from build123d import *

# Parameters (mm, degrees)
F0_R     = 53.975
F0_R_2   = 19.05
F0_R_3   = 12.7
F1_DEPTH = 12.7
F2_DEPTH = 50.8
F3_R     = 5.08
F4_SIZE  = 1.016


with BuildPart() as f1:
    # F0 (on Front) → F1 (new body)
    with BuildSketch(Plane.XZ):
        Circle(F0_R)
        with BuildLine():
            ThreePointArc((7.835162, 38.906399), (28.0633, 28.0633), (38.906399, 7.835162))
            ThreePointArc((38.906399, 7.835162), (44.971887, 5.837391), (47.5615, 0))
            ThreePointArc((47.5615, 0), (44.971887, -5.837391), (38.906399, -7.835162))
            ThreePointArc((38.906399, -7.835162), (28.0633, -28.0633), (7.835162, -38.906399))
            ThreePointArc((7.835162, -38.906399), (7.864284, -39.296467), (7.874, -39.6875))
            ThreePointArc((7.874, -39.6875), (-0.391033, -47.551784), (-7.835162, -38.906399))
            ThreePointArc((-7.835162, -38.906399), (-28.0633, -28.0633), (-38.906399, -7.835162))
            ThreePointArc((-38.906399, -7.835162), (-47.5615, 0), (-38.906399, 7.835162))
            ThreePointArc((-38.906399, 7.835162), (-28.0633, 28.0633), (-7.835162, 38.906399))
            ThreePointArc((-7.835162, 38.906399), (-0.391033, 47.551784), (7.874, 39.6875))
            ThreePointArc((7.874, 39.6875), (7.864284, 39.296467), (7.835162, 38.906399))
        make_face(mode=Mode.SUBTRACT)
        with BuildLine():
            ThreePointArc((38.906399, -7.835162), (31.8135, 0), (38.906399, 7.835162))
            ThreePointArc((38.906399, 7.835162), (28.0633, 28.0633), (7.835162, 38.906399))
            ThreePointArc((7.835162, 38.906399), (0, 31.8135), (-7.835162, 38.906399))
            ThreePointArc((-7.835162, 38.906399), (-28.0633, 28.0633), (-38.906399, 7.835162))
            ThreePointArc((-38.906399, 7.835162), (-33.850109, 5.284387), (-31.8135, 0))
            ThreePointArc((-31.8135, 0), (-33.850109, -5.284387), (-38.906399, -7.835162))
            ThreePointArc((-38.906399, -7.835162), (-28.0633, -28.0633), (-7.835162, -38.906399))
            ThreePointArc((-7.835162, -38.906399), (0, -31.8135), (7.835162, -38.906399))
            ThreePointArc((7.835162, -38.906399), (28.0633, -28.0633), (38.906399, -7.835162))
        make_face()
        Circle(F0_R_2, mode=Mode.SUBTRACT)
        Circle(F0_R_2)
        Circle(F0_R_3, mode=Mode.SUBTRACT)
    extrude(amount=F1_DEPTH)

    # F0 (on Front) → F2 (join)
    with BuildSketch(Plane.XZ):
        Circle(F0_R_2)
        Circle(F0_R_3, mode=Mode.SUBTRACT)
    extrude(amount=F2_DEPTH)

    # F3
    f3_edges = [f1.edges().sort_by_distance(p)[0] for p in [
        (-19.05, -12.7, 0),
    ]]
    fillet(f3_edges, radius=F3_R)

    # F4
    f4_edges = [f1.edges().sort_by_distance(p)[0] for p in [
        (53.975, -6.35, 0),
        (-53.975, 0, 0),
        (-53.975, -12.7, 0),
        (-40.468601, 0, -7.835162),
        (-38.906399, -6.35, 7.835162),
        (-40.468601, -12.7, -7.835162),
        (-7.835162, -6.35, -38.906399),
        (7.835162, 0, -40.468601),
        (7.835162, -12.7, -40.468601),
        (38.906399, -6.35, -7.835162),
        (40.468601, 0, 7.835162),
        (40.468601, -12.7, 7.835162),
        (7.874, -6.35, 39.6875),
        (-7.874, 0, 39.6875),
        (-7.874, -12.7, 39.6875),
        (-19.05, -50.8, 0),
        (-12.7, 0, 0),
        (12.7, -25.4, 0),
        (-12.7, -50.8, 0),
    ]]
    chamfer(f4_edges, length=F4_SIZE)


solid = f1.part
Input: part model. Units: mm. Frame: model coordinates. A direction names the side the tool comes from. Give positions to 0.01 mm unless a question says otherwise; leave off trailing zeros. Loops run counter-clockwise (first coordinate to the right, second up) from the corner with the lowest first, then second, coordinate; pieces in that order, holes last. Notation, with made-up numbers: (56, -29.5) -> (93, -29.5) arc R27 ccw to (93, -8.5) -> close; hole circle Ø3 at (45.5, 46). An arc over 180 degrees is marked (long way). Answer as a JSON object with one key per item and string values. Group by question number.
Item 1: Reachability of faces 1 (the cylindrical face through (-15.12, -33.56, -11.59)), 2 (the flat face through (12, -50.8, 7)) from +Z, -Z, +X, -X, +Y, -Y: full face, straight path, thin tool, end or side. Return the list, or none.
Item 2: Cut plane B-B, the plane z = 4. State how many separate pieces and enclosed holes the cut face has, and give its area (3 significant figures).
Item 3: Cut plane A-A, the plane y = -36.5. Return the cut outline in (x, z), and give its area (3 significant figures).
Item 4: Line query: probe 1 along Z at (x, y) = (0, -10.5) (1 decimal); probe 2 along Z at (x, y) = (-2, -10); probe 3 along Y at (x, z) = (-34.5, -31.5). Output: solid intervals per line, ascending.
Item 5: Pull-direction query (X, two-part tool) for faces 3 (the cylindrical face through (-39.78, -6.28, 36.48)), 4 (the cylindrical face through (-2.75, -25.06, -12.4)), 5 (the flat face through (11, 0, -11)); classes: released by +X, released by -X, zero draft, split by the parting line, or undercut.
Item 6: Pin query (flat end, axial travel): P1, Ø1.5, axis at y = -31, z = -14.5, coming from the +X side; P2, Ø2, axis at x = 11, y = -20, coming from the -Z side; P3, Ø4, axis at y = -24, z = 15.5, coming from the -X side; P4, Ø4, axis at x = -23.5, z = 6, coming from the +Y side. Return the tip coordinate at first contact, or that it passes through.
Checks:
{
 "1": {"face 1": "-Y", "face 2": "+Z, -Z, +X, -X, -Y"},
 "2": {"separate pieces": "4", "enclosed holes": "0", "area": "1,220 mm²"},
 "3": {"outline": "circle Ø38.1 at (0, 0); hole circle Ø25.4 at (0, 0)", "area": "633 mm²"},
 "4": {"probe 1": "z = -54 to -47.6, -31.8 to -12.7, 12.7 to 31.8, 47.6 to 54", "probe 2": "z = -53.94 to -47.3, -32.07 to -12.54, 12.54 to 32.07, 47.3 to 53.94", "probe 3": "y = -12.7 to 0"},
 "5": {"face 3": "split by the parting line", "face 4": "undercut", "face 5": "zero draft"},
 "6": {"P1": "stops at x = 13.18", "P2": "stops at z = -16.21", "P3": "stops at x = -13.44", "P4": "stops at y = 0"}
}
